Design review of the part shown in the three views and the two pictorial views. Dimensions are in mm from the part's minimum x, y and z. A direction names the side the tool comes from. Give positions to 0.01 mm unless a question says otherwise; leave off trailing zeros. Loops run counter-clockwise (first coordinate to the right, second up) from the corner with the lowest first, then second, coordinate; pieces in that order, holes last. Notation, with made-up numbers: (82, 83.5) - (130, 83.5) arc R10 cw to (130, 91.5) - close; hole circle Ø11 at (12, -32.75). An arc over 180 degrees is marked (long way). Answer in a Markdown table with one row per item.
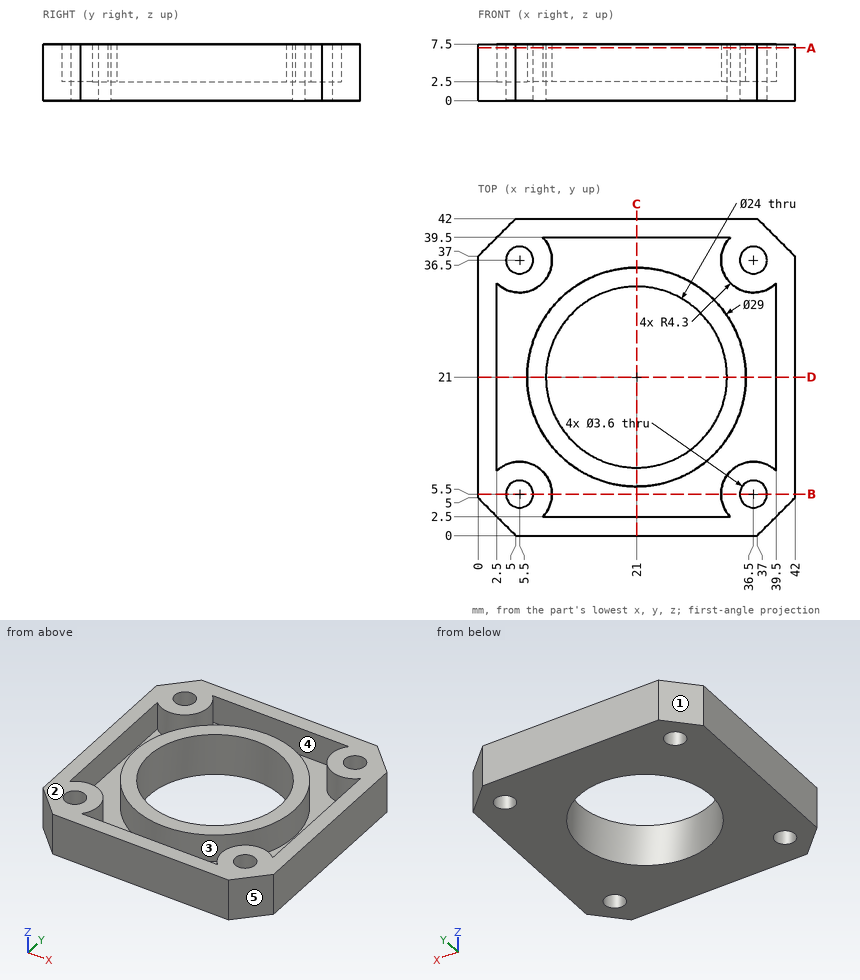
1. For the marked faces 4 and 5, list the 3-axis set-ups (+Z, -Z, +X, -X, +Y, -Y) from which the entire face can be reached by the end or side of a thin tool; tool diameter is ignored.
Values:
| item | result |
|---|---|
| face 4 | +Z |
| face 5 | +Z, -Z, +X, -Y |
2. Mouldability with a two-part tool opening along Y and no side actions: class the marked faces 1, 2 and 3 as released by +Y, released by -Y, zero draft, split by the parting line, or undercut.
Values:
| item | result |
|---|---|
| face 1 | released by +Y |
| face 2 | zero draft |
| face 3 | undercut |
3. Wall thickness on line 1 (Y direction, x = 5.5, z = 5); line 2 (X direction, y = 13, z = 7.25); line 3 (X direction, y = 4, z = 6.5): over which ranges is each line inside the solid? List them lowest first. Write a range as [from, to].
Values:
| item | result |
|---|---|
| line 1 | y = [0, 3.7], [7.3, 9.8], [32.2, 34.7], [38.3, 42] |
| line 2 | x = [0, 2.5], [8.91, 12.06], [29.94, 33.09], [39.5, 42] |
| line 3 | x = [1, 4.51], [6.49, 9.53], [32.47, 35.51], [37.49, 41] |
4. We need section C-C, the plane x = 21. Give the boundary of the cut face in (y, z), and give its area (3 significant figures).
Values:
| item | result |
|---|---|
| outline | (0, 0) - (9, 0) - (9, 7.5) - (6.5, 7.5) - (6.5, 2.5) - (2.5, 2.5) - (2.5, 7.5) - (0, 7.5) - close; (33, 0) - (42, 0) - (42, 7.5) - (39.5, 7.5) - (39.5, 2.5) - (35.5, 2.5) - (35.5, 7.5) - (33, 7.5) - close |
| area | 95.0 mm^2 |
5. We need section B-B, the plane y = 5.5. Give the boundary of the cut face in (x, z).
Values:
| item | result |
|---|---|
| outline | (0, 0) - (3.7, 0) - (3.7, 7.5) - (0, 7.5) - close; (7.3, 0) - (34.7, 0) - (34.7, 7.5) - (32.2, 7.5) - (32.2, 2.5) - (9.8, 2.5) - (9.8, 7.5) - (7.3, 7.5) - close; (38.3, 0) - (42, 0) - (42, 7.5) - (38.3, 7.5) - close |
6. We need section A-A, the plane z = 7. Give the boundary of the cut face in (x, y), and give its area (3 significant figures).
Values:
| item | result |
|---|---|
| outline | (0, 5) - (5, 0) - (37, 0) - (42, 5) - (42, 37) - (37, 42) - (5, 42) - (0, 37) - close; circle Ø29 at (21, 21); hole (2.5, 8.58) arc R4.3 cw to (8.58, 2.5) - (33.42, 2.5) arc R4.3 cw to (39.5, 8.58) - (39.5, 33.42) arc R4.3 cw to (33.42, 39.5) - (8.58, 39.5) arc R4.3 cw to (2.5, 33.42) - close; hole circle Ø3.6 at (5.5, 5.5); hole circle Ø3.6 at (5.5, 36.5); hole circle Ø24 at (21, 21); hole circle Ø3.6 at (36.5, 5.5); hole circle Ø3.6 at (36.5, 36.5) |
| area | 701 mm^2 |
